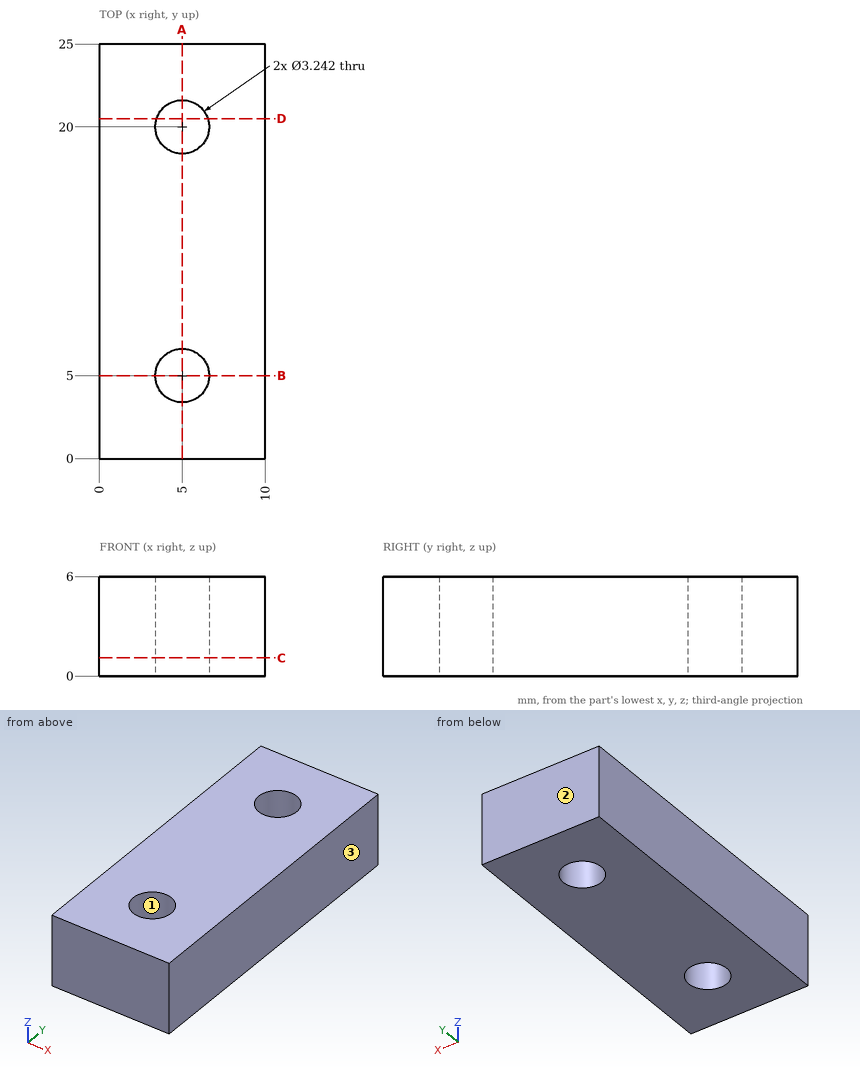
Geometry check sheet. Reference: drawing and pictorial views, mm from the part's lowest x, y, z. Give positions to 0.01 mm unless a question says otherwise; leave off trailing zeros. Order: outer loops, then holes, each group sorted by start corner. A loop starts at its lowest first (then second) coordinate and runs counter-clockwise, first axis right, second up. Notation, with made-up numbers: M -21.75,-7.5 L 32.25,-7.5 A21 ccw 32.25,27.5 Z; hole C -16.5,35.25 d5. An arc over 180 degrees is marked long. Answer as CSV lines item,"result". Start each with the question number.
Item 1: Mould release check, pull along X, two halves, no side actions. Record for the marked faces 1, 2 and 3: +X half, -X half, draft (parallel to the pull), parting line (faces both ways), or undercut.
Item 2: Cross-section at B-B on y = 5. Enter the section's corners in (x, z), plus the area to 3 significant figures.
Item 3: Thickness scan on line 1 (Y direction, x = 5, z = 3.45); line 2 (X direction, y = 5, z = 2.65); line 3 (Y direction, x = 5.75, z = 3.4). Record the ranges inside material, lowest first. Write a range as [from, to].
Item 4: Cross-section at C-C on z = 1.1. Enter the section's corners in (x, y).
Item 5: Cross-section at D-D on y = 20.5. Enter the section's corners in (x, z), plus the area to 3 significant figures.
Item 6: Cross-section at A-A on x = 5. Enter the section's corners in (y, z).
Established:
1,face 1,"undercut"
1,face 2,"draft"
1,face 3,"+X half"
2,outline,"M 0,0 L 3.38,0 L 3.38,6 L 0,6 Z; M 6.62,0 L 10,0 L 10,6 L 6.62,6 Z"
2,area,"40.5 mm^2"
3,line 1,"y = [0, 3.38], [6.62, 18.38], [21.62, 25]"
3,line 2,"x = [0, 3.38], [6.62, 10]"
3,line 3,"y = [0, 3.56], [6.44, 18.56], [21.44, 25]"
4,outline,"M 0,0 L 10,0 L 10,25 L 0,25 Z; hole C 5,5 d3.24; hole C 5,20 d3.24"
5,outline,"M 0,0 L 3.46,0 L 3.46,6 L 0,6 Z; M 6.54,0 L 10,0 L 10,6 L 6.54,6 Z"
5,area,"41.5 mm^2"
6,outline,"M 0,0 L 3.38,0 L 3.38,6 L 0,6 Z; M 6.62,0 L 18.38,0 L 18.38,6 L 6.62,6 Z; M 21.62,0 L 25,0 L 25,6 L 21.62,6 Z"
